from build123d import *

# Parameters (mm, degrees)
BOSS_EXTRU_1_DEPTH           = 50
ENL_V_MAT_EXTRU_1_DEPTH      = 78.151108828
ENL_V_MAT_EXTRU_1_DEPTH_BACK = 78.151108828
ESQUISSE2_W                  = 42
ESQUISSE2_H                  = 27.125696421
ESQUISSE2_H_2                = 2.874303579


with BuildPart() as part:
    # Esquisse1 → Boss.-Extru.1 (new body)
    with BuildSketch(Plane.XY):
        with BuildLine():
            Line((-2, -28.65), (-2, -9.797958971))
            ThreePointArc((-2, -9.797958971), (-7.745966692, -6.32455532), (-10, 0))
            add(Edge.make_bspline(
                [(-10, 0), (-10.038102543, -9.915248827), (-2.132148039, -18.010708935), (-2, -28.65)],
                knots=[0, 0, 0, 0, 1, 1, 1, 1], degree=3))
        make_face()
        with BuildLine():
            Line((3, -17.125696421), (3, -9.539392014))
            ThreePointArc((3, -9.539392014), (0.516443819, -9.986655385), (-2, -9.797958971))
            Line((-2, -9.797958971), (-2, -28.65))
            Line((-2, -28.65), (-2, -57.3))
            Line((-2, -57.3), (3, -57.3))
            Line((3, -57.3), (3, -17.125696421))
        make_face()
        with BuildLine():
            ThreePointArc((9.937144604, -1.119445002), (7.717920999, -6.358749519), (3, -9.539392014))
            Line((3, -9.539392014), (3, -17.125696421))
            add(Edge.make_bspline(
                [(9.937144604, -1.119445002), (9.273451903, -8.836768249), (4.143675796, -10.613482839), (3, -17.125696421)],
                knots=[0.044553807, 0.044553807, 0.044553807, 0.044553807, 1, 1, 1, 1], degree=3))
        make_face()
        with BuildLine():
            ThreePointArc((-2, -1.5), (-0.790569415, 2.371708245), (2.5, 0))
            Line((2.5, 0), (3, 0))
            Line((3, 0), (3, -9.539392014))
            ThreePointArc((3, -9.539392014), (7.717920999, -6.358749519), (9.937144604, -1.119445002))
            add(Edge.make_bspline(
                [(10, 0), (9.989331014, -0.386787822), (9.968093534, -0.759575306), (9.937144604, -1.119445002)],
                knots=[0, 0, 0, 0, 0.044553807, 0.044553807, 0.044553807, 0.044553807], degree=3))
            ThreePointArc((10, 0), (0, 10), (-10, 0))
            ThreePointArc((-10, 0), (-7.745966692, -6.32455532), (-2, -9.797958971))
            Line((-2, -9.797958971), (-2, -1.5))
        make_face()
        with BuildLine():
            Line((3, 0), (2.5, 0))
            ThreePointArc((2.5, 0), (0.790569415, -2.371708245), (-2, -1.5))
            Line((-2, -1.5), (-2, -9.797958971))
            ThreePointArc((-2, -9.797958971), (0.516443819, -9.986655385), (3, -9.539392014))
            Line((3, -9.539392014), (3, 0))
        make_face()
    extrude(amount=BOSS_EXTRU_1_DEPTH)

    # Esquisse2 → Enl_v. mat.-Extru.1 (cut, two sides: drawn at the far end of the back side and taken through both)
    with BuildSketch(Plane(origin=(3, 0, 0), x_dir=(0, 0, -1), z_dir=(1, 0, 0)).offset(-ENL_V_MAT_EXTRU_1_DEPTH_BACK)):
        with BuildLine():
            add(Edge.make_bspline(
                [(-4, -20), (-8.708547212, -27.751388753), (-14.537623568, -36.046397597), (-25, -37.3)],
                knots=[0, 0, 0, 0, 1, 1, 1, 1], degree=3))
            add(Edge.make_bspline(
                [(-46, -20), (-40.775649876, -29.315136052), (-33.796978395, -35.093732661), (-25, -37.3)],
                knots=[0, 0, 0, 0, 1, 1, 1, 1], degree=3))
            Line((-46, -20), (-4, -20))
        make_face()
        with Locations((-25, -3.562848211)):
            Rectangle(ESQUISSE2_W, ESQUISSE2_H)
        with Locations((-25, -18.562848211)):
            Rectangle(ESQUISSE2_W, ESQUISSE2_H_2)
        with BuildLine():
            Line((-50, -57.3), (-35, -57.3))
            Line((-35, -57.3), (-35, -47.3))
            add(Edge.make_bspline(
                [(-35, -47.3), (-35.073971228, -43.269856006), (-36.614804988, -40.092663019), (-38.683033976, -37.3)],
                knots=[0, 0, 0, 0, 0.317822392, 0.317822392, 0.317822392, 0.317822392], degree=3))
            Line((-38.683033976, -37.3), (-46, -37.3))
            Line((-46, -37.3), (-46, -29.06189571))
            add(Edge.make_bspline(
                [(-46, -29.06189571), (-48.274731382, -26.370504837), (-49.995661884, -23.543129972), (-50, -20)],
                knots=[0.658761608, 0.658761608, 0.658761608, 0.658761608, 1, 1, 1, 1], degree=3))
            Line((-50, -20), (-50, -57.3))
        make_face()
        with BuildLine():
            Line((-15, -47.3), (-15, -57.3))
            Line((-15, -57.3), (0, -57.3))
            Line((0, -57.3), (0, -17.125696421))
            add(Edge.make_bspline(
                [(-4, -29.937309986), (-1.817418752, -26.399450919), (-0.142614882, -22.257986482), (0, -17.125696421)],
                knots=[0.670508014, 0.670508014, 0.670508014, 0.670508014, 1, 1, 1, 1], degree=3))
            Line((-4, -29.937309986), (-4, -37.3))
            Line((-4, -37.3), (-9.549596223, -37.3))
            add(Edge.make_bspline(
                [(-15, -47.3), (-14.991223802, -43.931361101), (-12.499880822, -40.852999709), (-9.549596223, -37.3)],
                knots=[0, 0, 0, 0, 0.413424981, 0.413424981, 0.413424981, 0.413424981], degree=3))
        make_face()
        with BuildLine():
            add(Edge.make_bspline(
                [(-9.549596223, -37.3), (-7.714999508, -35.090612608), (-5.702938557, -32.697691357), (-4, -29.937309986)],
                knots=[0.413424981, 0.413424981, 0.413424981, 0.413424981, 0.670508014, 0.670508014, 0.670508014, 0.670508014], degree=3))
            Line((-9.549596223, -37.3), (-4, -37.3))
            Line((-4, -37.3), (-4, -29.937309986))
        make_face()
        with BuildLine():
            Line((-46, -37.3), (-38.683033976, -37.3))
            add(Edge.make_bspline(
                [(-38.683033976, -37.3), (-40.901695677, -34.304212532), (-43.727262954, -31.750926947), (-46, -29.06189571)],
                knots=[0.317822392, 0.317822392, 0.317822392, 0.317822392, 0.658761608, 0.658761608, 0.658761608, 0.658761608], degree=3))
            Line((-46, -29.06189571), (-46, -37.3))
        make_face()
    extrude(amount=ENL_V_MAT_EXTRU_1_DEPTH + ENL_V_MAT_EXTRU_1_DEPTH_BACK, mode=Mode.SUBTRACT)


solid = part.part
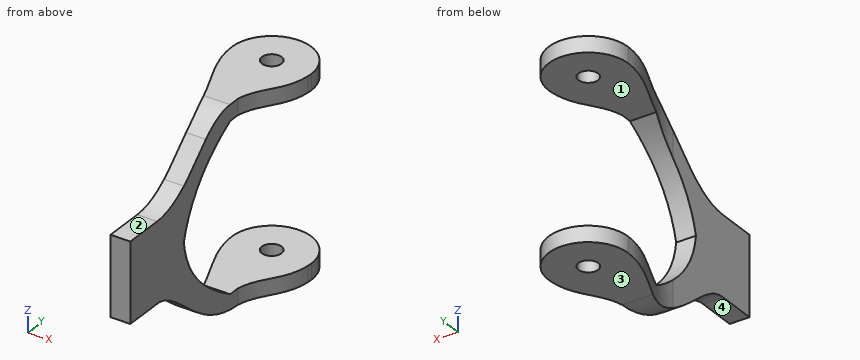
Verification items for the finished model (mm, model axes). Face numbers are marked on the shaded views. A direction names the side the tool comes from. Give positions to 0.01 mm unless a question says otherwise; leave off trailing zeros.
(1) Gauge pin test, flat ends, axial feed: pin 1 (8 mm diameter, centred on x = 0, y = 0, fed in from -Z); pin 2 (5.5 mm diameter, centred on x = 0, y = -51.5, fed in from -Z); pin 3 (23 mm diameter, centred on y = -46, z = 29.5, fed in from -X); pin 4 (3 mm diameter, centred on x = 1, y = -40, fed in from +Z). Record the tip position at first contact, or that the pin passes through.
(2) Material ranges on line 1 (Z direction, x = -3.25, y = -15.5); line 2 (Y direction, x = 0, z = 47.1); line 3 (Y direction, x = 0, z = 48.1), recorded low to high.
(3) Access from +Z, -Z, +X, -X, +Y, -Y to the whole of each face (thin tool, end or side, straight path). Record for the marked faces 1, 2, 3 and 4.
(4) Cross-section at A-A (x = 0). State how many separate pieces and enclosed holes the cut face has, plus the area to 3 significant figures.
Worked out:
1. pin 1: stops at z = 0
1. pin 2: stops at z = 15
1. pin 3: stops at x = -2
1. pin 4: stops at z = 37.85
2. line 1: z = 0 to 4, 46 to 50
2. line 2: y = -27.68 to -2.5, 2.5 to 10
2. line 3: y = -26.22 to -2.5, 2.5 to 10
3. face 1: +X, -X, +Y
3. face 2: +Z, +X, -X, -Y
3. face 3: -Z, +X, -X, +Y, -Y
3. face 4: -Z, +X, -X, -Y
4. separate pieces: 3
4. enclosed holes: 0
4. area: 880 mm2
